Geometry check sheet. Reference: the model listing, model coordinates, mm. Round coordinates to 2 decimals unless told otherwise and drop trailing zeros. Order: outer loops, then holes, each group sorted by start corner. A loop starts at its lowest first (then second) coordinate and runs counter-clockwise, first axis right, second up. Notation, with made-up numbers: (-13.5, -23) - (22.5, -23) arc R27 ccw to (22.5, 14) - close; hole circle Ø1 at (51, 17.25). An arc over 180 degrees is marked (long way). Return JSON: item names as keys, results as strings. Group by question number.
Q1. Sectioned sample at C-C, the plane y = -2. Record the cut outline in (x, z).
Q2. Sectioned sample at B-B, the plane z = -19.05. Record the cut outline in (x, y), then the cut area to 3 significant figures.
Q3. Material ranges on line 1 along X through (y, z) = (-1.25, -19.5); line 2 along X through (y, z) = (1, -40); line 3 along X through (y, z) = (2, -97), recorded low to high.
Q4. Gauge pin test, flat ends, axial feed: pin 1 Ø10 at (x, z) = (127, -19.05) entering from -Y; pin 2 Ø3 at (x, y) = (21, 0) entering from +Z; pin 3 Ø3 at (y, z) = (-2.5, -40) entering from -X; pin 4 Ø5 at (x, y) = (84, 1) entering from +Z. Record the tip position at first contact, or that the pin passes through.
Q5. Sectioned sample at D-D, the plane x = 101.6. Record the cut outline in (y, z).
Q6. Sectioned sample at A-A, the plane x = 19.05. Record the cut outline in (y, z).
```python
from build123d import *

# Parameters (mm, degrees)
SKETCH1_W                = 146.05
SKETCH1_H                = 146.05
BOSS_EXTRUDE1_DEPTH      = 4.7625
SKETCH2_R                = 6.477
SKETCH2_R_2              = 2.19075
CUT_EXTRUDE1_DEPTH       = 207.765399971
S_0_348_DIAMETER_HOLE1_D = 8.8392
CUT_EXTRUDE2_DEPTH       = 207.765399971
FILLET1_R                = 12.7
FILLET2_R                = 50.8


with BuildPart() as part:
    # Sketch1 → Boss-Extrude1 (new, symmetric)
    with BuildSketch(Plane(origin=(0, 0, 0), x_dir=(1, 0, 0), z_dir=(0, 1, 0))):
        with Locations((73.025, 73.025)):
            Rectangle(SKETCH1_W, SKETCH1_H)
    extrude(amount=BOSS_EXTRUDE1_DEPTH, both=True)

    # Sketch2 → Cut-Extrude1 (cut, through all)
    with BuildSketch(Plane(origin=(0, 4.7625, 0), x_dir=(1, 0, 0), z_dir=(0, 1, 0))):
        with Locations(Location((101.6, 101.6, 0), (0, 0, 270))):
            Circle(SKETCH2_R)
        with Locations(Location((101.6, 91.28125, 0), (0, 0, 270))):
            Circle(SKETCH2_R_2)
        with Locations(Location((101.6, 111.91875, 0), (0, 0, 270))):
            Circle(SKETCH2_R_2)
    extrude(amount=-CUT_EXTRUDE1_DEPTH, mode=Mode.SUBTRACT)

    # S (0.348) Diameter Hole1 (through all)
    with Locations(Plane(origin=(0, 4.7625, 0), x_dir=(1, 0, 0), z_dir=(0, 1, 0))):
        with Locations((19.05, 127), (127, 19.05), (57.15, 19.05), (19.05, 57.15)):
            Hole(S_0_348_DIAMETER_HOLE1_D / 2)

    # Sketch5 → Cut-Extrude2 (cut, through all)
    with BuildSketch(Plane(origin=(0, 4.7625, 0), x_dir=(1, 0, 0), z_dir=(0, 1, 0))):
        with BuildLine():
            Line((0, 107.95), (38.1, 107.95))
            ThreePointArc((38.1, 107.95), (87.491408666, 87.491408666), (107.95, 38.1))
            Line((107.95, 38.1), (107.95, 0))
            Line((107.95, 0), (0, 0))
            Line((0, 0), (0, 107.95))
        make_face()
    extrude(amount=-CUT_EXTRUDE2_DEPTH, mode=Mode.SUBTRACT)

    # Fillet1
    fillet1_edges = [part.edges().sort_by_distance(p)[0] for p in [
        (0, 0, -107.95),
        (107.95, 0, 0),
        (0, 0, -146.05),
        (146.05, 0, 0),
    ]]
    fillet(fillet1_edges, radius=FILLET1_R)

    # Fillet2
    fillet2_edges = [part.edges().sort_by_distance(p)[0] for p in [
        (146.05, 0, -146.05),
    ]]
    fillet(fillet2_edges, radius=FILLET2_R)


solid = part.part
```
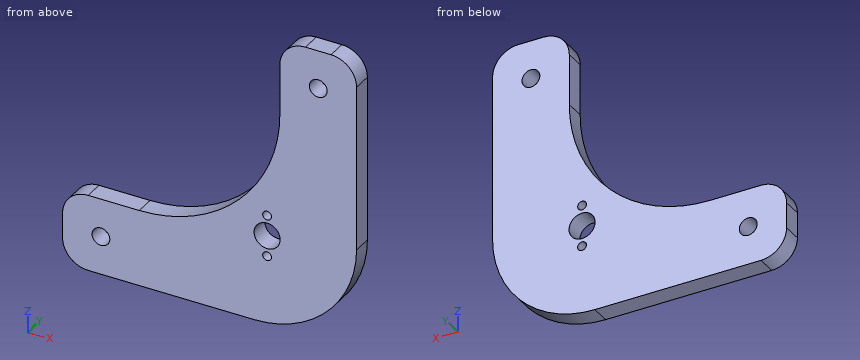
Reply:
{
 "1": {"outline": "(0, -133.35) arc R12.7 ccw to (12.7, -146.05) - (95.25, -146.05) arc R50.8 ccw to (146.05, -95.25) - (146.05, -12.7) arc R12.7 ccw to (133.35, 0) - (120.65, 0) arc R12.7 ccw to (107.95, -12.7) - (107.95, -38.1) arc R69.85 cw to (38.1, -107.95) - (12.7, -107.95) arc R12.7 ccw to (0, -120.65) - close; hole circle Ø8.84 at (19.05, -127); hole circle Ø12.95 at (101.6, -101.6); hole circle Ø4.38 at (101.6, -111.92); hole circle Ø4.38 at (101.6, -91.28); hole circle Ø8.84 at (127, -19.05)"},
 "2": {"outline": "(107.95, -4.76) - (122.58, -4.76) - (122.58, 4.76) - (107.95, 4.76) - close; (131.42, -4.76) - (146.05, -4.76) - (146.05, 4.76) - (131.42, 4.76) - close", "area": "279 mm^2"},
 "3": {"line 1": "107.95 to 122.6, 131.4 to 146.05", "line 2": "107.92 to 146.05", "line 3": "75.65 to 97.04, 106.16 to 146.02"},
 "4": {"pin 1": "y = -4.76", "pin 2": "z = -107.95", "pin 3": "x = 107.87", "pin 4": "z = -88.46"},
 "5": {"outline": "(-4.76, -145.65) - (4.76, -145.65) - (4.76, -114.11) - (-4.76, -114.11) - close; (-4.76, -109.73) - (4.76, -109.73) - (4.76, -108.08) - (-4.76, -108.08) - close; (-4.76, -95.12) - (4.76, -95.12) - (4.76, -93.47) - (-4.76, -93.47) - close; (-4.76, -89.09) - (4.76, -89.09) - (4.76, -67.2) - (-4.76, -67.2) - close"},
 "6": {"outline": "(-4.76, -146.05) - (4.76, -146.05) - (4.76, -131.42) - (-4.76, -131.42) - close; (-4.76, -122.58) - (4.76, -122.58) - (4.76, -107.95) - (-4.76, -107.95) - close"}
}
